Can you work these out from the model? Positions are in its coordinate system, mm. Round coordinates to 2 decimals unless told otherwise and drop trailing zeros. Write each loop counter-clockwise with the first axis right and the second up, starting at its lowest first coordinate (ties: lowest second). Pieces come first, ordered by that corner, then holes.
Q1. If we section it at D-D (y = -11.25): Please give me the cut outline in (x, z).
Q2. If we section it at C-C (y = 22.5): Please give me the cut outline in (x, z).
Q3. We'd pull the mould along X, two halves only. Please class faces 1 (the cylindrical face through (-8.67, -39.05, 0.49)), 2 (the cylindrical face through (20.871, -11.825, 0.507)), 3 (the flat face through (-1, 9, 0)): +X half, -X half, draft (parallel to the pull), parting line (faces both ways), or undercut.
Q4. Please list where these lines run through material, in increasing order: line 1 along X through (y, z) = (2.5, 0.15); line 2 along X through (y, z) = (-8, 0.7); line 3 along Y through (x, z) = (7, 0.6).
Q5. I'm going to push a flat-ended pin straight in: pin 1 Ø1.8 at (x, y) = (0, 22.5) entering from -Z. Where does the tip first touch, or does it pass through?
Q6. If we section it at B-B (x = -7): Please give me the cut outline in (y, z), plus the area to 3 significant figures.
Q7. If we section it at A-A (z = 0.2): Give the number of separate pieces and of enclosed holes in the cut face, plus the area to 3 significant figures.
from build123d import *

# Parameters (mm, degrees)
SKETCH_1_R          = 40
SKETCH_1_R_2        = 2.5
SKETCH_1_R_3        = 1.5
EXTRUDE_1_DEPTH     = 1
SKETCH_2_R          = 1.5
CUT_EXTRUDE_1_DEPTH = 10
SKETCH_3_R          = 3
CUT_EXTRUDE_2_DEPTH = 10


with BuildPart() as part:
    # 草图1 → 凸台-拉伸1 (new body)
    with BuildSketch(Plane.XY):
        Circle(SKETCH_1_R)
        Circle(SKETCH_1_R_2, mode=Mode.SUBTRACT)
        with Locations((0, 7)):
            Circle(SKETCH_1_R_3, mode=Mode.SUBTRACT)
        with Locations((7, 0)):
            Circle(SKETCH_1_R_3, mode=Mode.SUBTRACT)
        with Locations((0, -7)):
            Circle(SKETCH_1_R_3, mode=Mode.SUBTRACT)
        with Locations((-7, 0)):
            Circle(SKETCH_1_R_3, mode=Mode.SUBTRACT)
    extrude(amount=EXTRUDE_1_DEPTH)

    # 草图2 → 切除-拉伸1 (cut)
    with BuildSketch(Plane.XY.offset(1)):
        with Locations((0, 22.5)):
            Circle(SKETCH_2_R)
        with Locations((19.485571585, -11.25)):
            Circle(SKETCH_2_R)
        with Locations((-19.485571585, -11.25)):
            Circle(SKETCH_2_R)
    extrude(amount=-CUT_EXTRUDE_1_DEPTH, mode=Mode.SUBTRACT)

    # 草图3 → 切除-拉伸2 (cut)
    with BuildSketch(Plane.XY.offset(1)):
        Circle(SKETCH_3_R)
    extrude(amount=-CUT_EXTRUDE_2_DEPTH, mode=Mode.SUBTRACT)


solid = part.part
A:
1. outline: (-38.39, 0) - (-20.99, 0) - (-20.99, 1) - (-38.39, 1) - close; (-17.99, 0) - (17.99, 0) - (17.99, 1) - (-17.99, 1) - close; (20.99, 0) - (38.39, 0) - (38.39, 1) - (20.99, 1) - close
2. outline: (-33.07, 0) - (-1.5, 0) - (-1.5, 1) - (-33.07, 1) - close; (1.5, 0) - (33.07, 0) - (33.07, 1) - (1.5, 1) - close
3. face 1: parting line
3. face 2: undercut
3. face 3: draft
4. line 1: x = -39.92 to -1.66, 1.66 to 39.92
4. line 2: x = -39.19 to -1.12, 1.12 to 39.19
4. line 3: y = -39.38 to -1.5, 1.5 to 39.38
5. pin 1: passes through
6. outline: (-39.38, 0) - (-1.5, 0) - (-1.5, 1) - (-39.38, 1) - close; (1.5, 0) - (39.38, 0) - (39.38, 1) - (1.5, 1) - close
6. area: 75.8 mm2
7. separate pieces: 1
7. enclosed holes: 8
7. area: 4,950 mm2
